Geometry: final body of the model. Coordinates: model frame, mm. A direction names the side the tool comes from. Coordinates: 2 decimals unless noted, no trailing zeros. Order: outer loops, then holes, each group sorted by start corner. A loop starts at its lowest first (then second) coordinate and runs counter-clockwise, first axis right, second up. Notation, with made-up numbers: M 18,84 L 42,84 A18 cw 42,117 Z; hole C 47,55 d4. An arc over 180 degrees is marked long. One line per question, with ' | ' between items.
from build123d import *

# Parameters (mm, degrees)
F1_DEPTH = 63.5
F0_W     = 25.4
F0_H     = 19.05
F2_DEPTH = 25.4
F3_DEPTH = 7.9375
F0_W_2   = 11.0026748776
F0_H_2   = 28.575
F5_R     = 6.35


with BuildPart() as f1:
    # F0 (on Front) → F1 (new body, symmetric)
    with BuildSketch(Plane.XZ):
        Polygon((22.225, 9.525), (-41.275, 9.525), (-41.275, -9.525), (41.275, -9.525), (41.275, 9.525), align=None)
    extrude(amount=F1_DEPTH, both=True)

    # F0 (on Front) → F2 (join, symmetric)
    with BuildSketch(Plane.XZ):
        with BuildLine():
            Line((22.225, 27.0002), (22.225, 9.525))
            Line((22.225, 9.525), (41.275, 9.525))
            Line((41.275, 9.525), (41.275, 27.0002))
            ThreePointArc((41.275, 27.0002), (45.9246798487, 38.2255201513), (57.15, 42.8752))
            Line((57.15, 42.8752), (60.325, 42.8752))
            Line((60.325, 42.8752), (60.325, 61.9252))
            Line((60.325, 61.9252), (57.15, 61.9252))
            ThreePointArc((57.15, 61.9252), (32.4542956671, 51.6959043329), (22.225, 27.0002))
        make_face()
        with Locations((73.025, 52.4002)):
            Rectangle(F0_W, F0_H)
    extrude(amount=F2_DEPTH, both=True)

    # F0 (on Front) → F3 (join, symmetric)
    with BuildSketch(Plane.XZ):
        with BuildLine():
            add(Edge.make_bspline(
                [(-41.275, 9.525), (-41.275, 29.0701329026), (12.5299637369, 61.9252), (57.15, 61.9252)],
                knots=[0, 0, 0, 0, 111.5045361635, 111.5045361635, 111.5045361635, 111.5045361635], degree=3))
            Line((-41.275, 9.525), (22.225, 9.525))
            Line((22.225, 9.525), (22.225, 27.0002))
            ThreePointArc((22.225, 27.0002), (32.4542956671, 51.6959043329), (57.15, 61.9252))
        make_face()
    extrude(amount=F3_DEPTH, both=True)

    # F0 (on Front) → F4 (revolve)
    with BuildSketch(Plane.XZ):
        with Locations((105.6236625612, 52.3875)):
            Rectangle(F0_W_2, F0_H_2)
    revolve(axis=Axis((85.725, 0, 52.3875), (0, 0, 1)))

    # F5
    f5_edges = [f1.edges().sort_by_distance(p)[0] for p in [
        (-41.275, -63.5, 0),
        (41.275, -63.5, 0),
        (41.275, 63.5, 0),
        (-41.275, 63.5, 0),
    ]]
    fillet(f5_edges, radius=F5_R)

    # F0 (on Front) → F6 (revolve, cut)
    with BuildSketch(Plane.XZ):
        Polygon((85.725, 66.675), (85.725, 61.9252), (85.725, 42.8752), (85.725, 38.1), (100.1223251224, 38.1), (100.1223251224, 66.675), align=None)
    revolve(axis=Axis((85.725, 0, 52.3875), (0, 0, 1)), mode=Mode.SUBTRACT)


solid = f1.part
1. Access query for faces 4 (the face through (46, 25.4, 42)), 5 (the face through (-2, -7.938, 30)), 6 (the face through (22.225, 17, 18)), 7 (the face through (45.8, -0.4, 38.1)), 8 (the face through (41.275, -1, 4)). Directions: +Z, -Z, +X, -X, +Y, -Y. A direction counts if a zero-diameter tool reaches every point of the face in a straight line with its end or side. Return the directions, or none.
Response values:
face 4: +Z, +X, -X, +Y | face 5: +Z, -X, -Y | face 6: +Z, -X, +Y | face 7: -Z, +Y, -Y | face 8: -Z, +X, +Y, -Y
2. Section A-A, the plane y = -37. Output: boundary loops of the cut face in (x, z) (3 decimals), and give its area (3 significant figures).
Response values:
outline: M -41.275,-9.525 L 41.275,-9.525 L 41.275,9.525 L -41.275,9.525 Z | area: 1,570 mm^2
3. Material intervals for line 1 (Y direction, x = 86.5, z = 53.5); line 2 (Z direction, x = 13.5, y = -19.5) (3 decimals); line 3 (Y direction, x = 67, z = 45.5), sorted ascending. Write a range as [from, to].
Response values:
line 1: y = [-25.39, -14.38], [14.38, 25.39] | line 2: z = [-9.525, 9.525] | line 3: y = [-25.4, 25.4]
4. Pin query (flat end, axial travel): P1, Ø14.5, axis at x = 65, y = 9, coming from the -Z side; P2, Ø16.5, axis at x = 1, y = 43, coming from the +Z side (3 decimals); P3, Ø8, axis at x = 40, z = 54, coming from the +Y side. Return the tip coordinate at first contact, or that it passes through.
Response values:
P1: stops at z = 38.1 | P2: stops at z = 9.525 | P3: stops at y = 25.4
5. Draft query along X for faces 1 (the face through (-2, 7.938, 30)), 2 (the face through (74.3, -8.76, 52.59)), 3 (the face through (32.73, -16.79, 51.97)). Return one class per face: pulls with the +X half, pulls with the -X half, needs draft (parallel to the pull), parting line crosses it, or undercut.
Response values:
face 1: needs draft | face 2: undercut | face 3: pulls with the -X half
